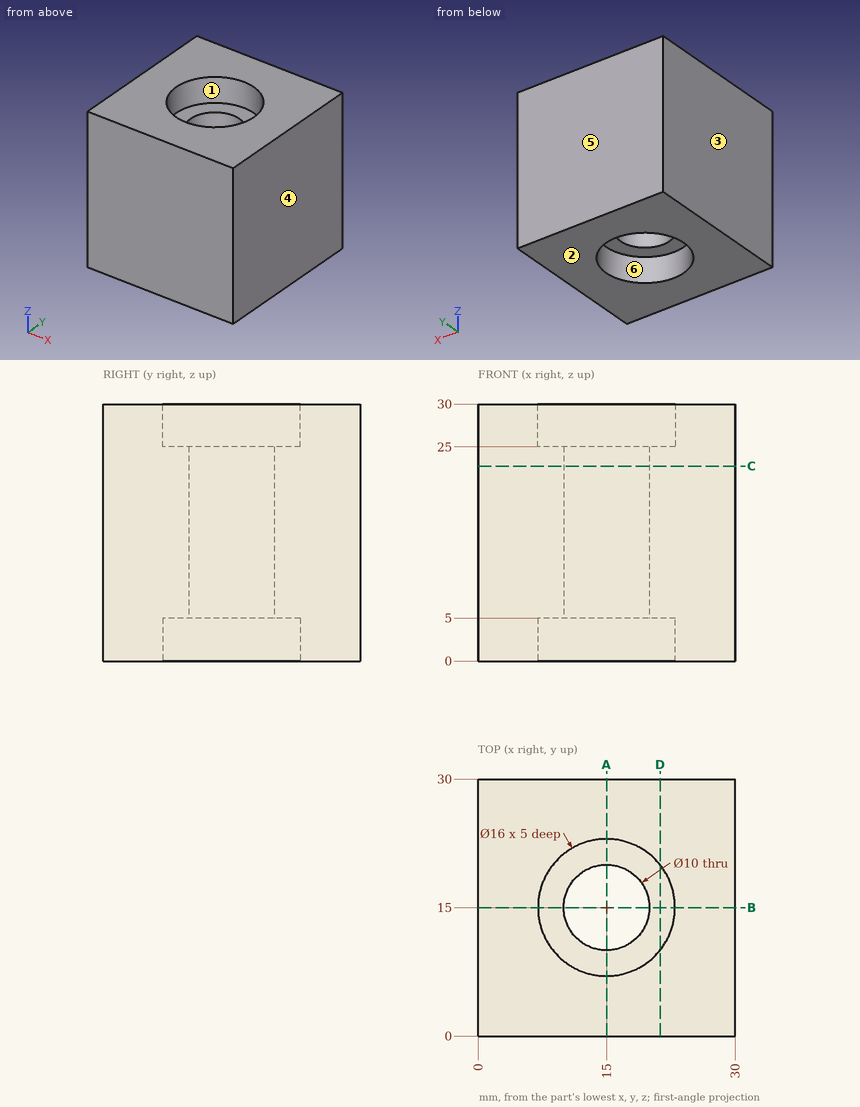
Job drawing, mm, ordinate dimensions from the low corner. One solid piece. A direction names the side the tool comes from. Round coordinates to 2 decimals unless told otherwise and drop trailing zeros. Write each loop counter-clockwise with the first axis right and the second up, starting at its lowest first coordinate (ties: lowest second). Pieces come first, ordered by that corner, then holes. Notation, with made-up numbers: (62, -33.75) -> (121, -33.75) arc R23 cw to (121, -21.75) -> close; hole circle Ø5 at (9.25, 13.5). An arc over 180 degrees is marked (long way). Answer as a JSON object with one key per item and string values.
(1) Two-plate mould, pull along X, no slides. Class the marked faces 1, 2, 3 and 4: +X half, -X half, draft (parallel to the pull), parting line (faces both ways), or undercut.
Reported:
{"face 1": "undercut", "face 2": "draft", "face 3": "-X half", "face 4": "+X half"}
(2) Probe probe 1 along Y at (x, z) = (15, 27.45); probe 2 along X at (y, z) = (8.75, 4.75); probe 3 along Z at (x, y) = (15.25, 8.5). List the from-to ranges inside material, lowest first. Write a range as [from, to].
Reported:
{"probe 1": "y = [0, 7], [23, 30]", "probe 2": "x = [0, 10.01], [19.99, 30]", "probe 3": "z = [5, 25]"}
(3) Band-saw the part on D-D, the plane x = 21.25. List the corners of the cut face in (y, z).
Reported:
{"outline": "(0, 0) -> (10.01, 0) -> (10.01, 5) -> (19.99, 5) -> (19.99, 0) -> (30, 0) -> (30, 30) -> (19.99, 30) -> (19.99, 25) -> (10.01, 25) -> (10.01, 30) -> (0, 30) -> close"}
(4) Band-saw the part on A-A, the plane x = 15. List the corners of the cut face in (y, z), then the cut area to 3 significant figures.
Reported:
{"outline": "(0, 0) -> (7, 0) -> (7, 5) -> (10, 5) -> (10, 25) -> (7, 25) -> (7, 30) -> (0, 30) -> close; (20, 5) -> (23, 5) -> (23, 0) -> (30, 0) -> (30, 30) -> (23, 30) -> (23, 25) -> (20, 25) -> close", "area": "540 mm^2"}
(5) Pin check, flat tips, straight feed: P1, Ø5, axis at x = 18, y = 16.5, coming from the -Z side; P2, Ø4, axis at x = 3.5, z = 7.5, coming from the -Y side. Stop position of each tip, or through.
Reported:
{"P1": "stops at z = 5", "P2": "stops at y = 0"}
(6) Which spindle directions (+Z, -Z, +X, -X, +Y, -Y) get a long thin tool onto all of the face, cutting with end or side? Do the marked faces 5 and 6. Say none if no direction does.
Reported:
{"face 5": "+Z, -Z, +X, -X, +Y", "face 6": "-Z"}
(7) Band-saw the part on C-C, the plane z = 22.75. List the corners of the cut face in (x, y), then the cut area to 3 significant figures.
Reported:
{"outline": "(0, 0) -> (30, 0) -> (30, 30) -> (0, 30) -> close; hole circle Ø10 at (15, 15)", "area": "821 mm^2"}
